Geometry: final body of the model. Coordinates: model frame, mm. Give positions to 0.01 mm unless a question says otherwise; leave off trailing zeros. Write each loop counter-clockwise with the first axis right and the second up, starting at its lowest first coordinate (ties: lowest second). Pieces come first, ordered by that corner, then holes. Notation, with made-up numbers: (-22, -4.5) -> (-15, -4.5) arc R11 cw to (-15, 5.5) -> close; hole circle Ø6 at (59.25, 73.5). An arc over 180 degrees is marked (long way). Answer as a JSON object with one key per item and string values.
from build123d import *

# Parameters (mm, degrees)
SKETCH_W              = 115
SKETCH_H              = 25
PAD_DEPTH             = 3
PAD001_DEPTH          = 3
SKETCH002_W           = 115
SKETCH002_H           = 25
SKETCH002_W_2         = 96
SKETCH002_H_2         = 3
PAD002_DEPTH          = 3
SKETCH003_R           = 1.55
POCKET_DEPTH          = 245.060315
POLARPATTERN_COUNT    = 2
POLARPATTERN001_COUNT = 2
POLARPATTERN002_COUNT = 2
FILLET_R              = 2


with BuildPart() as part:
    # Sketch → Pad (new body)
    with BuildSketch(Plane.XY):
        Rectangle(SKETCH_W, SKETCH_H)
    extrude(amount=PAD_DEPTH)

    # Sketch001 (on Face6 of Pad) → Pad001 (join)
    with BuildSketch(Plane.XY.offset(3)):
        Polygon((-57.5, 12.5), (57.5, 12.5), (57.5, 4), (50, 4), (50, 5), (-50, 5), (-50, 4), (-57.5, 4), align=None)
        Polygon((-57.5, -12.5), (57.5, -12.5), (57.5, -4), (50, -4), (50, -5), (-50, -5), (-50, -4), (-57.5, -4), align=None)
    extrude(amount=PAD001_DEPTH)

    # Sketch002 (on Face12 of Pad001) → Pad002 (join)
    with BuildSketch(Plane.XY.offset(6)):
        Rectangle(SKETCH002_W, SKETCH002_H)
        Rectangle(SKETCH002_W_2, SKETCH002_H_2, mode=Mode.SUBTRACT)
    extrude(amount=PAD002_DEPTH)

    # Sketch003 (on Face26 of Pad002) → Pocket (cut, through all)
    with BuildSketch(Plane.XY.offset(9)):
        with Locations((-52.5, 7.5)):
            Circle(SKETCH003_R)
    pocket = extrude(amount=-POCKET_DEPTH, mode=Mode.SUBTRACT)

    # PolarPattern: Pocket ×2 about axis
    polarpattern_axis = Axis((0, 0, 0), (0, 1, 0))
    for i in range(1, POLARPATTERN_COUNT):
        add(pocket.rotate(polarpattern_axis, i * 360 / POLARPATTERN_COUNT), mode=Mode.SUBTRACT)

    # PolarPattern001: Pocket ×2 about axis
    polarpattern001_axis = Axis((0, 0, 0), (1, 0, 0))
    for i in range(1, POLARPATTERN001_COUNT):
        add(pocket.rotate(polarpattern001_axis, i * 360 / POLARPATTERN001_COUNT), mode=Mode.SUBTRACT)

    # PolarPattern002: Pocket ×2 about axis
    polarpattern002_axis = Axis((0, 0, 9), (0, 0, 1))
    for i in range(1, POLARPATTERN002_COUNT):
        add(pocket.rotate(polarpattern002_axis, i * 360 / POLARPATTERN002_COUNT), mode=Mode.SUBTRACT)

    # Fillet
    fillet_edges = [part.edges().sort_by_distance(p)[0] for p in [
        (57.5, 12.5, 7.5),
        (57.5, 12.5, 4.5),
        (57.5, 12.5, 1.5),
        (57.5, -12.5, 7.5),
        (-57.5, 12.5, 7.5),
        (-57.5, -12.5, 7.5),
    ]]
    fillet(fillet_edges, radius=FILLET_R)


solid = part.part
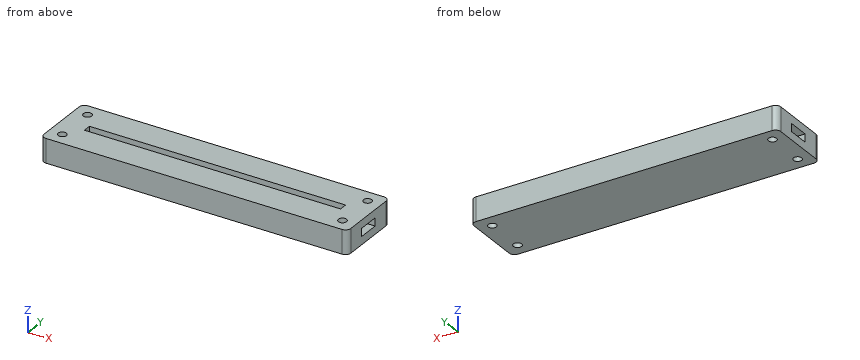
Q1. Cut plane A-A (x = -52.5). Return the cut outline in (y, z).
Values:
{"outline": "(-12.5, 0) -> (-9.05, 0) -> (-9.05, 9) -> (-12.5, 9) -> close; (-5.95, 0) -> (5.95, 0) -> (5.95, 9) -> (-5.95, 9) -> close; (9.05, 0) -> (12.5, 0) -> (12.5, 9) -> (9.05, 9) -> close; hole (-4, 3) -> (4, 3) -> (4, 6) -> (-4, 6) -> close"}
Q2. Material intervals for L1, parallel to Y at x = 52.5, z = 3.25; L2, parallel to X at y = -7.5, z = 3; L3, parallel to Z at x = 45, y = 2.75, sorted ascending. Write a range as from..to.
Values:
{"L1": "-12.5..-9.05, -5.95..-4, 4..5.95, 9.05..12.5", "L2": "-57.5..-54.05, -50.95..50.95, 54.05..57.5", "L3": "0..3, 6..9"}
Q3. Cut plane D-D (x = 0.5). Return the cut outline in (y, z), and give its area (3 significant figures).
Values:
{"outline": "(-12.5, 0) -> (12.5, 0) -> (12.5, 9) -> (1.5, 9) -> (1.5, 6) -> (5, 6) -> (5, 3) -> (-5, 3) -> (-5, 6) -> (-1.5, 6) -> (-1.5, 9) -> (-12.5, 9) -> close", "area": "186 mm²"}
Q4. Cut plane C-C (y = 7.5). Return the cut outline in (x, z).
Values:
{"outline": "(-57.5, 0) -> (-54.05, 0) -> (-54.05, 9) -> (-57.5, 9) -> close; (-50.95, 0) -> (50.95, 0) -> (50.95, 9) -> (-50.95, 9) -> close; (54.05, 0) -> (57.5, 0) -> (57.5, 9) -> (54.05, 9) -> close"}
Q5. Cut plane B-B (z = 4). Return the cut outline in (x, y).
Values:
{"outline": "(-57.5, -10.5) arc R2 ccw to (-55.5, -12.5) -> (55.5, -12.5) arc R2 ccw to (57.5, -10.5) -> (57.5, -4) -> (50, -4) -> (50, -5) -> (-50, -5) -> (-50, -4) -> (-57.5, -4) -> close; (-57.5, 4) -> (-50, 4) -> (-50, 5) -> (50, 5) -> (50, 4) -> (57.5, 4) -> (57.5, 10.5) arc R2 ccw to (55.5, 12.5) -> (-55.5, 12.5) arc R2 ccw to (-57.5, 10.5) -> close; hole circle Ø3.1 at (-52.5, -7.5); hole circle Ø3.1 at (-52.5, 7.5); hole circle Ø3.1 at (52.5, -7.5); hole circle Ø3.1 at (52.5, 7.5)"}
Q6. First-contact query: P1, Ø1.9, axis at x = -52.5, y = 7.5, coming from the +Z side; P2, Ø1.5, axis at x = 18, y = 0.5, coming from the +Z side. Flat tips, straight axial feed; report the tip coordinate or a pass-through.
Values:
{"P1": "through", "P2": "z = 3"}
